Input: part model. Units: mm. Frame: model coordinates. Face numbers are marked on the shaded views. A direction names the side the tool comes from. Give positions to 0.01 mm unless a question says otherwise; leave off trailing zeros. Loops run counter-clockwise (first coordinate to the right, second up) from the corner with the lowest first, then second, coordinate; pieces in that order, holes last. Notation, with made-up numbers: (70.25, 3.5) -> (94.25, 3.5) arc R24 cw to (94.25, 23.5) -> close; hole circle Ø3 at (9.25, 58.25). An arc over 180 degrees is marked (long way). Answer as a JSON object with one key per item and string values. Group by question number.
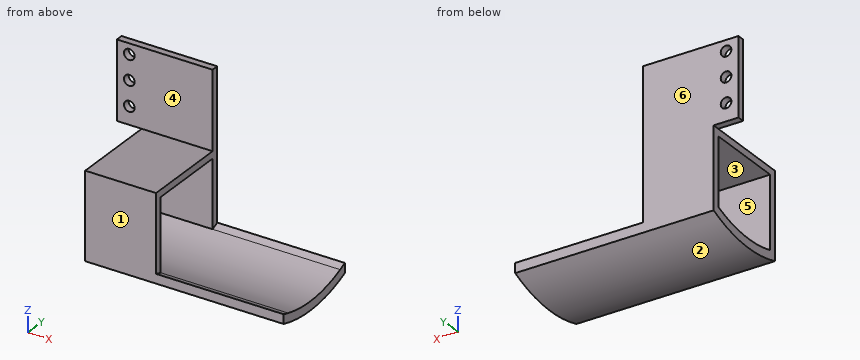
```python
from build123d import *

# Parameters (mm, degrees)
SKETCH3_W           = 27
SKETCH3_H           = 22
SKETCH3_R           = 1.5
BOSS_EXTRUDE5_DEPTH = 2
BOSS_EXTRUDE6_DEPTH = 20
BOSS_EXTRUDE7_DEPTH = 56


with BuildPart() as part:
    # Sketch3 → Boss-Extrude5 (new body)
    with BuildSketch(Plane(origin=(0, 13.2, 0), x_dir=(1, 0, 0), z_dir=(0, 1, 0))):
        with Locations((34.5, 60.85)):
            Rectangle(SKETCH3_W, SKETCH3_H)
        with Locations((24.5, 59.85)):
            Circle(SKETCH3_R, mode=Mode.SUBTRACT)
        with Locations((24.5, 66.85)):
            Circle(SKETCH3_R, mode=Mode.SUBTRACT)
        with Locations((24.5, 52.85)):
            Circle(SKETCH3_R, mode=Mode.SUBTRACT)
    extrude(amount=BOSS_EXTRUDE5_DEPTH)

    # Sketch4 → Boss-Extrude6 (add)
    with BuildSketch(Plane.ZY.offset(-28)):
        Polygon((-71.85, -11.2), (-71.85, 15.2), (-73.85, 15.2), (-73.85, 13.2), (-73.85, -9.2), (-73.85, -11.2), align=None)
        with BuildLine():
            Line((-73.85, 13.2), (-73.85, 15.2))
            Line((-73.85, 15.2), (-92.027131173, 15.2))
            ThreePointArc((-92.027131173, 15.2), (-92.486915012, 14.206944358), (-92.915428425, 13.2))
            Line((-92.915428425, 13.2), (-73.85, 13.2))
        make_face()
        with BuildLine():
            Line((-93.659613991, -11.2), (-73.85, -11.2))
            Line((-73.85, -11.2), (-73.85, -9.2))
            Line((-73.85, -9.2), (-94.269216751, -9.2))
            ThreePointArc((-94.269216751, -9.2), (-93.979353281, -10.204553096), (-93.659613991, -11.2))
        make_face()
    extrude(amount=-BOSS_EXTRUDE6_DEPTH)

    # Sketch4_3 → Boss-Extrude7 (add)
    with BuildSketch(Plane.ZY.offset(-28)):
        with BuildLine():
            ThreePointArc((-92.915428425, 13.2), (-92.486915012, 14.206944358), (-92.027131173, 15.2))
            Line((-92.027131173, 15.2), (-94.78133603, 15.2))
            ThreePointArc((-94.78133603, 15.2), (-97.939046263, 2.137244706), (-96.288405944, -11.2))
            Line((-96.288405944, -11.2), (-93.659613991, -11.2))
            ThreePointArc((-93.659613991, -11.2), (-93.979353281, -10.204553096), (-94.269216751, -9.2))
            ThreePointArc((-94.269216751, -9.2), (-95.436253581, 2.111441618), (-92.915428425, 13.2))
        make_face()
    extrude(amount=-BOSS_EXTRUDE7_DEPTH)


solid = part.part
```
Q1. Set-up query: the marked faces 4, 5 and 6. Return all of +Z, -Z, +X, -X, +Y, -Y with unobstructed straight access to the full face (end or side cutting, diameter ignored); none if empty.
Q2. Pull-direction query (Y, two-part tool) for the marked faces 1, 2 and 3; classes: +Y half, -Y half, draft (parallel to the pull), parting line (faces both ways), or undercut.
Q3. Section D-D on y = -2.75. Return the cut outline in (x, z), then the cut area to 3 significant figures.
Q4. Pin query (flat end, axial travel): pin 1 Ø13 at (y, z) = (7, -79.5) entering from -X; pin 2 Ø2 at (x, z) = (50.5, -77) entering from +Y; pin 3 Ø1 at (x, y) = (53, 5.5) entering from -Z; pin 4 Ø3.5 at (x, z) = (24.5, -52.85) entering from +Y. Return the tip coordinate at first contact, or that it passes through.
Q5. Ray query, probe 1 along Z at (x, y) = (24.5, 14.85); probe 2 along Y at (x, z) = (41, -88); probe 3 along X at (y, z) = (13.9, -52.85). Return the intervals inside material, ascending.
Q6. Section A-A on z = -52.85. Return the cut outline in (x, y), then the cut area to 3 significant figures.
Q7. Section C-C on x = 44. Return the cut outline in (y, z).
Q8. Section B-B on x = 24.5. Return the cut outline in (y, z), then the cut area to 3 significant figures.
Numbers:
{
 "1": {"face 4": "+Z, +X, -X, -Y", "face 5": "+X, -X", "face 6": "+Z, -Z, +X, -X, +Y"},
 "2": {"face 1": "-Y half", "face 2": "parting line", "face 3": "undercut"},
 "3": {"outline": "(28, -97.9) -> (84, -97.9) -> (84, -95.39) -> (28, -95.39) -> close; (28, -73.85) -> (48, -73.85) -> (48, -71.85) -> (28, -71.85) -> close", "area": "180 mm²"},
 "4": {"pin 1": "stops at x = 28", "pin 2": "passes through", "pin 3": "stops at z = -97.67", "pin 4": "stops at y = 15.2"},
 "5": {"probe 1": "z = -71.85 to -68.35, -65.35 to -61.35, -58.35 to -54.35, -51.35 to -49.85", "probe 2": "y = -11.2 to -9.2, 13.2 to 15.2", "probe 3": "x = 21 to 23, 26 to 48"},
 "6": {"outline": "(21, 13.2) -> (23, 13.2) -> (23, 15.2) -> (21, 15.2) -> close; (26, 13.2) -> (48, 13.2) -> (48, 15.2) -> (26, 15.2) -> close", "area": "48.0 mm²"},
 "7": {"outline": "(-11.2, -96.29) arc R37.5 ccw to (15.2, -94.78) -> (15.2, -49.85) -> (13.2, -49.85) -> (13.2, -71.85) -> (-11.2, -71.85) -> close; hole (-9.2, -94.27) arc R35 ccw to (13.2, -92.92) -> (13.2, -73.85) -> (-9.2, -73.85) -> close"},
 "8": {"outline": "(13.2, -71.85) -> (15.2, -71.85) -> (15.2, -68.35) -> (13.2, -68.35) -> close; (13.2, -65.35) -> (15.2, -65.35) -> (15.2, -61.35) -> (13.2, -61.35) -> close; (13.2, -58.35) -> (15.2, -58.35) -> (15.2, -54.35) -> (13.2, -54.35) -> close; (13.2, -51.35) -> (15.2, -51.35) -> (15.2, -49.85) -> (13.2, -49.85) -> close", "area": "26.0 mm²"}
}
